Autodesk Inventor part; units mm, degrees
ref_plane "Work Plane1" through (0, 0, -80) normal (0, 0, -1) x (-1, 0, 0)
ref_plane "YZ Plane" through (0, 0, 0) normal (1, 0, 0) x (0, 1, 0)
ref_plane "XZ Plane" through (0, 0, 0) normal (0, 1, 0) x (-1, 0, 0)
sketch "Sketch1" plane through (0, 0, 0) normal (0, 0, 1) x (1, 0, 0)
  circle A0 centre (0, 0) radius 9.5
  line L0 (70, 35) -> (80, 35)
  line L1 (80, 35) -> (80, -35)
  line L2 (80, -35) -> (70, -35)
  line L3 (70, -35) -> (70, 35)
  line L4 (70, 35) -> (80, -35) construction
  line L5 (80, 35) -> (70, -35) construction
  arc A1 (-3.4517, 24.7606) -> (-3.4517, -24.7606) centre (0, 0) ccw
  line L6 (70, 35) -> (-3.4517, 24.7606)
  line L7 (70, -35) -> (-3.4517, -24.7606)
  line L8 (0, 0) -> (70, 0)
  point P0 (75, 0)
  dimension "d0" = 19
  dimension "d11" = 10
  dimension "d12" = 70
  dimension "d13" = 50
  dimension "d25" = 70
extrude "Extrusion1" add sketch "Sketch1" along normal blind 10
ref_plane "Work Plane1" through (0, 0, -80) normal (0, 0, -1) x (-1, 0, 0)
sketch "Sketch2" plane through (0, 0, -80) normal (0, 0, -1) x (-1, 0, 0)
  circle A0 centre (0, 0) radius 9.5
  arc A1 (3.4517, -24.7606) -> (3.4517, 24.7606) centre (0, 0) ccw
  line L0 (-70, 35) -> (3.4517, 24.7606)
  line L1 (-80, 35) -> (-70, 35)
  line L2 (-80, -35) -> (-80, 35)
  line L3 (-70, -35) -> (-80, -35)
  line L4 (3.4517, -24.7606) -> (-70, -35)
  circle A2 centre (0, 0) radius 9.5
extrude "Extrusion2" add sketch "Sketch2" along normal blind 10
extrude "Extrusion3" add sketch "Sketch1" against normal blind 80 contours L3 L0 L1 L2
sketch "Sketch3" plane through (80, -35, 10) normal (1, 0, 0) x (0, 0, -1)
  line L0 (0, 0) -> (0, 70) construction
  line L1 (0, 70) -> (100, 0) construction
  line L2 (100, 0) -> (0, 0)
  line L3 (15, 70) -> (85, 70)
  line L4 (85, 70) -> (85, 0)
  line L5 (85, 0) -> (15, 0)
  line L6 (15, 0) -> (15, 70)
  line L7 (15, 70) -> (85, 0) construction
  line L8 (85, 70) -> (15, 0) construction
  line L9 (25, 60) -> (75, 60)
  line L10 (75, 60) -> (75, 10)
  line L11 (75, 10) -> (25, 10)
  line L12 (25, 10) -> (25, 60)
  line L13 (25, 60) -> (75, 10) construction
  line L14 (75, 60) -> (25, 10) construction
  point P0 (10, 35)
  point P1 (50, 35)
  point P2 (50, 35)
  point P3 (15, 0)
  point P4 (160, 0)
  dimension "d14" = 70
  dimension "d15" = 50
  dimension "d16" = 50
extrude "Extrusion4" add sketch "Sketch3" along normal blind 30
sketch "Sketch4" plane through (70, 35, -75) normal (0, 0, -1) x (1, 0, 0)
  line L0 (10, 0) -> (40, 0) construction
  line L1 (40, 70) -> (40, 0) construction
  line L2 (10, 0) -> (40, 70) construction
  line L3 (25, 35) -> (25, 50) construction
  line L4 (25, 50) -> (25, 20) construction
  circle A0 centre (25, 50) radius 2
  circle A1 centre (25, 20) radius 2
  point P0 (-70, 35)
  dimension "d19" = 15
  dimension "d20" = 30
  dimension "d21" = 4
  dimension "d22" = 4
extrude "Extrusion5" cut sketch "Sketch4" against normal blind 70
properties part number "Forearm-End Fork" material "Acrylic, Clear"
Geometry: final body of the model. Coordinates: model frame, mm. A direction names the side the tool comes from. Give positions to 0.01 mm unless a question says otherwise; leave off trailing zeros. Loops run counter-clockwise (first coordinate to the right, second up) from the corner with the lowest first, then second, coordinate; pieces in that order, holes last. Notation, with made-up numbers: M 69,14.25 L 89,14.25 A15 cw 89,23.25 Z; hole C 2,3 d5. An arc over 180 degrees is marked long. Put each result on its own line as item: value. Start each with the question number.
1) Cut plane A-A (x = 95). Output: boundary loops of the cut face in (y, z).
2) Cut plane C-C (z = 1.5). Output: boundary loops of the cut face in (x, y).
3) Cut plane B-B (y = 0). Output: boundary loops of the cut face in (x, z).
4) Access query for faces 4 (the flat face through (95, 25, -40)), 5 (the flat face through (90, 35, -39)), 6 (the flat face through (70, 0, -39)), 7 (the flat face through (80, 0, -82)), 8 (the flat face through (95, 0, -5)). Directions: +Z, -Z, +X, -X, +Y, -Y. A direction counts if a zero-diameter tool reaches every point of the face in a straight line with its end or side. Return the directions, or none.
5) Ray query, line 1 along Y through (x, z) = (95, -69); line 2 along Z through (x, y) = (57, 12.5); line 3 along Z through (x, y) = (100, 9.5). Return the intervals inside material, ascending.
6) Cut plane D-D (x = 36.5). Output: boundary loops of the cut face in (y, z).
7) Pull-direction query (X, two-part tool) for faces 1 (the flat face through (95, 0, -15)), 2 (the cylindrical face through (-24.995, 0.501, -84.93)), 3 (the cylindrical face through (96.908, 14.399, -10.07)); classes: pulls with the +X half, pulls with the -X half, needs draft (parallel to the pull), parting line crosses it, or undercut.
8) Contact query for flat-ended pins moving along their axis: pin 1 (1 mm diameter, centred on y = 9, z = -71, fed in from -X); pin 2 (6.5 mm diameter, centred on x = 95, y = 15, fed in from -Z); pin 3 (15 mm diameter, centred on x = 95, y = 9.5, fed in from +Z); pin 4 (3 mm diameter, centred on x = 95, y = -15, fed in from -Z). Output: stop coordinate, or through.
Verdict:
1. outline: M -35,-75 L -17,-75 L -17,-65 L -25,-65 L -25,-15 L -17,-15 L -17,-5 L -35,-5 Z; M -13,-75 L 13,-75 L 13,-65 L -13,-65 Z; M -13,-15 L 13,-15 L 13,-5 L -13,-5 Z; M 17,-75 L 35,-75 L 35,-5 L 17,-5 L 17,-15 L 25,-15 L 25,-65 L 17,-65 Z
2. outline: M -3.45,-24.76 L 70,-35 L 80,-35 L 80,35 L 70,35 L -3.45,24.76 A25 ccw Z; hole C 0,0 d19
3. outline: M -25,-90 L -9.5,-90 L -9.5,-80 L -25,-80 Z; M -25,0 L -9.5,0 L -9.5,10 L -25,10 Z; M 9.5,-90 L 80,-90 L 80,-75 L 110,-75 L 110,-65 L 80,-65 L 80,-15 L 110,-15 L 110,-5 L 80,-5 L 80,10 L 9.5,10 L 9.5,0 L 70,0 L 70,-80 L 9.5,-80 Z
4. face 4: +X
4. face 5: +Z, -Z, +X, -X, +Y
4. face 6: -X, +Y, -Y
4. face 7: -Z, +X, +Y, -Y
4. face 8: +Z, +X, +Y, -Y
5. line 1: -35 to -17, -13 to 13, 17 to 35
5. line 2: -90 to -80, 0 to 10
5. line 3: -75 to -65, -15 to -5
6. outline: M -30.33,-90 L 30.33,-90 L 30.33,-80 L -30.33,-80 Z; M -30.33,0 L 30.33,0 L 30.33,10 L -30.33,10 Z
7. face 1: needs draft
7. face 2: pulls with the -X half
7. face 3: undercut
8. pin 1: x = 70
8. pin 2: z = -75
8. pin 3: z = -5
8. pin 4: through
